Geometry: see drawing. Coordinates: mm, zero at the bounding-box minimum. Round coordinates to 2 decimals unless told otherwise and drop trailing zeros. Order: outer loops, then holes, each group sorted by start corner. A loop starts at its lowest first (then second) coordinate and runs counter-clockwise, first axis right, second up. Notation, with made-up numbers: (-22.75, 72) - (-12.75, 72) arc R11 ccw to (-12.75, 77) - close; hole circle Ø2 at (72, -36). An arc over 180 degrees is marked (long way). Put each result on its own line as item: value. Start each with the question number.
1) Section D-D on x = 12.7. Output: boundary loops of the cut face in (y, z) (1 decimal), then the cut area to 3 significant figures.
2) Section C-C on z = 2.4. State how many separate pieces and enclosed holes the cut face has, then the cut area to 3 significant figures.
3) Line query: probe 1 along Y at (x, z) = (38.1, 0.9); probe 2 along X at (y, z) = (37, 1.3) (1 decimal); probe 3 along Y at (x, z) = (39, 2.9) (1 decimal). Output: solid intervals per line, ascending. Write a range as [from, to].
4) Section A-A on y = 38.1. Output: boundary loops of the cut face in (x, z) (1 decimal).
5) Section B-B on x = 38.1. Output: boundary loops of the cut face in (y, z) (1 decimal), then the cut area to 3 significant figures.
6) Contact query for a flat-ended pin moving along its axis: P1, Ø1, axis at x = 13, z = 2, coming from the -Y side (1 decimal). Output: stop coordinate, or through.
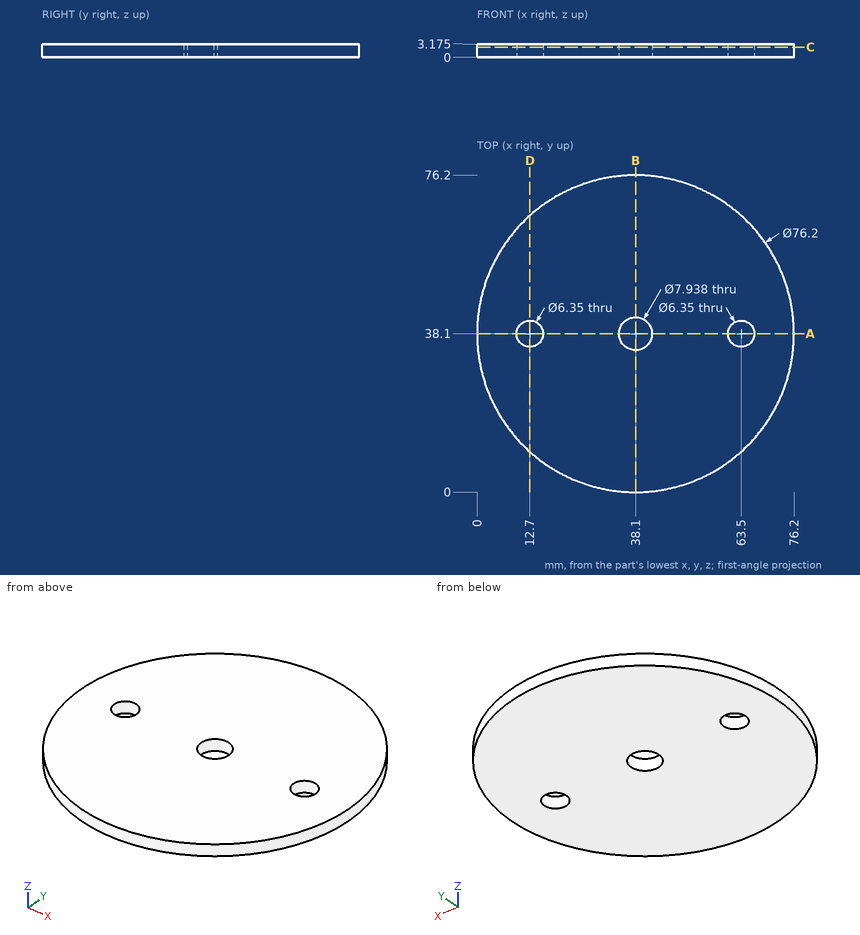
Answer sheet:
1. outline: (9.7, 0) - (34.9, 0) - (34.9, 3.2) - (9.7, 3.2) - close; (41.3, 0) - (66.5, 0) - (66.5, 3.2) - (41.3, 3.2) - close
1. area: 160 mm^2
2. separate pieces: 1
2. enclosed holes: 3
2. area: 4,450 mm^2
3. probe 1: [0, 34.13], [42.07, 76.2]
3. probe 2: [0, 9.7], [15.7, 34.3], [41.9, 60.5], [66.5, 76.2]
3. probe 3: [0, 34.2], [42, 76.2]
4. outline: (0, 0) - (9.5, 0) - (9.5, 3.2) - (0, 3.2) - close; (15.9, 0) - (34.1, 0) - (34.1, 3.2) - (15.9, 3.2) - close; (42.1, 0) - (60.3, 0) - (60.3, 3.2) - (42.1, 3.2) - close; (66.7, 0) - (76.2, 0) - (76.2, 3.2) - (66.7, 3.2) - close
5. outline: (0, 0) - (34.1, 0) - (34.1, 3.2) - (0, 3.2) - close; (42.1, 0) - (76.2, 0) - (76.2, 3.2) - (42.1, 3.2) - close
5. area: 217 mm^2
6. P1: y = 9
